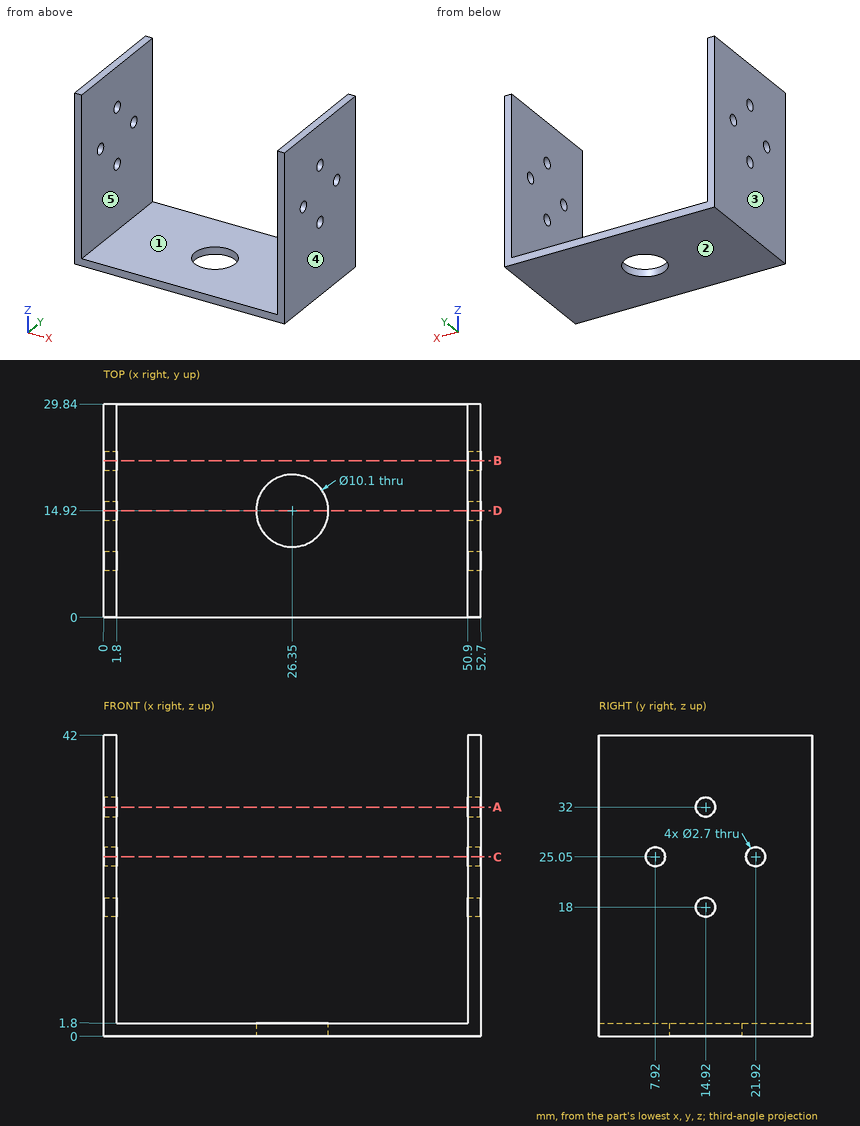
Geometry check sheet. Reference: drawing and pictorial views, mm from the part's lowest x, y, z. A direction names the side the tool comes from. Give positions to 0.01 mm unless a question says otherwise; leave off trailing zeros. Order: outer loops, then holes, each group sorted by start corner. A loop starts at its lowest first (then second) coordinate and runs counter-clockwise, first axis right, second up.
1. Access from +Z, -Z, +X, -X, +Y, -Y to the whole of each face (thin tool, end or side, straight path). Record for the marked faces 1 and 2.
2. Thickness scan on L1, parallel to Y at x = 52, z = 25.05; L2, parallel to X at y = 21.5, z = 39; L3, parallel to Y at x = 26.35, z = 1.1. Record the ranges inside material, lowest first.
3. Section check B-B, the plane y = 21.92. Enter the section's corners in (x, z), and give its area (3 significant figures).
4. Section check A-A, the plane z = 32. Enter the section's corners in (x, y).
5. Section check D-D, the plane y = 14.92. Enter the section's corners in (x, z), and give its area (3 significant figures).
6. Section check C-C, the plane z = 25.05. Enter the section's corners in (x, y), and give its area (3 significant figures).
7. Release check for a two-part mould opening along X. For the marked faces 3, 4 and 5 record: pulls with the +X half, pulls with the -X half, needs draft (parallel to the pull), parting line crosses it, or undercut.
Values follow:
1. face 1: +Z, +Y, -Y
1. face 2: -Z, +X, -X, +Y, -Y
2. L1: y = 0 to 6.57, 9.27 to 20.57, 23.27 to 29.84
2. L2: x = 0 to 1.8, 50.9 to 52.7
2. L3: y = 0 to 9.87, 19.97 to 29.84
3. outline: (0, 0) - (52.7, 0) - (52.7, 23.7) - (50.9, 23.7) - (50.9, 1.8) - (1.8, 1.8) - (1.8, 23.7) - (0, 23.7) - close; (0, 26.4) - (1.8, 26.4) - (1.8, 42) - (0, 42) - close; (50.9, 26.4) - (52.7, 26.4) - (52.7, 42) - (50.9, 42) - close
3. area: 230 mm2
4. outline: (0, 0) - (1.8, 0) - (1.8, 13.57) - (0, 13.57) - close; (0, 16.27) - (1.8, 16.27) - (1.8, 29.84) - (0, 29.84) - close; (50.9, 0) - (52.7, 0) - (52.7, 13.57) - (50.9, 13.57) - close; (50.9, 16.27) - (52.7, 16.27) - (52.7, 29.84) - (50.9, 29.84) - close
5. outline: (0, 0) - (21.3, 0) - (21.3, 1.8) - (1.8, 1.8) - (1.8, 16.65) - (0, 16.65) - close; (0, 19.35) - (1.8, 19.35) - (1.8, 30.65) - (0, 30.65) - close; (0, 33.35) - (1.8, 33.35) - (1.8, 42) - (0, 42) - close; (31.4, 0) - (52.7, 0) - (52.7, 16.65) - (50.9, 16.65) - (50.9, 1.8) - (31.4, 1.8) - close; (50.9, 19.35) - (52.7, 19.35) - (52.7, 30.65) - (50.9, 30.65) - close; (50.9, 33.35) - (52.7, 33.35) - (52.7, 42) - (50.9, 42) - close
5. area: 202 mm2
6. outline: (0, 0) - (1.8, 0) - (1.8, 6.57) - (0, 6.57) - close; (0, 9.27) - (1.8, 9.27) - (1.8, 20.57) - (0, 20.57) - close; (0, 23.27) - (1.8, 23.27) - (1.8, 29.84) - (0, 29.84) - close; (50.9, 0) - (52.7, 0) - (52.7, 6.57) - (50.9, 6.57) - close; (50.9, 9.27) - (52.7, 9.27) - (52.7, 20.57) - (50.9, 20.57) - close; (50.9, 23.27) - (52.7, 23.27) - (52.7, 29.84) - (50.9, 29.84) - close
6. area: 88.0 mm2
7. face 3: pulls with the -X half
7. face 4: pulls with the +X half
7. face 5: undercut
